from build123d import *

# Parameters (mm, degrees)
SKETCH1_W            = 694
SKETCH1_H            = 693
BOSS_EXTRUDE1_DEPTH  = 3
M6_CLEARANCE_HOLE1_D = 6.6
LPATTERN1_COUNT      = 3
LPATTERN1_PITCH      = 297
MIRROR1_COPY_1_D     = 6.6
MIRROR1_COPY_2_D     = 6.6
M6_CLEARANCE_HOLE2_D = 6.6
LPATTERN2_COUNT      = 2
LPATTERN2_PITCH      = 293
MIRROR2_COPY_1_D     = 6.6
FILLET1_R            = 10
SKETCH6_R            = 4
SKETCH6_R_2          = 5
SKETCH6_R_3          = 15
CUT_EXTRUDE1_DEPTH   = 4


with BuildPart() as part:
    # Sketch1 → Boss-Extrude1 (new body)
    with BuildSketch(Plane(origin=(0, 0, 0), x_dir=(1, 0, 0), z_dir=(0, 1, 0))):
        Rectangle(SKETCH1_W, SKETCH1_H)
    extrude(amount=BOSS_EXTRUDE1_DEPTH)

    # M6 Clearance Hole1 (through all)
    with Locations(Plane(origin=(0, 3, 0), x_dir=(1, 0, 0), z_dir=(0, 1, 0))):
        with Locations((297, -337.5)):
            m6_clearance_hole1 = Hole(M6_CLEARANCE_HOLE1_D / 2)

    # LPattern1: M6 Clearance Hole1 ×3
    with Locations(*[(-i * LPATTERN1_PITCH, 0, 0) for i in range(1, LPATTERN1_COUNT)]):
        add(m6_clearance_hole1, mode=Mode.SUBTRACT)

    # Mirror1: M6 Clearance Hole1 across plane
    add(m6_clearance_hole1.mirror(Plane.XY), mode=Mode.SUBTRACT)

    # Mirror1 copy 1 (through all)
    with Locations(Plane(origin=(-297, 3, 0), x_dir=(1, 0, 0), z_dir=(0, 1, 0))):
        with Locations((297, 337.5)):
            Hole(MIRROR1_COPY_1_D / 2)

    # Mirror1 copy 2 (through all)
    with Locations(Plane(origin=(-594, 3, 0), x_dir=(1, 0, 0), z_dir=(0, 1, 0))):
        with Locations((297, 337.5)):
            Hole(MIRROR1_COPY_2_D / 2)

    # M6 Clearance Hole2 (through all)
    with Locations(Plane(origin=(0, 3, 0), x_dir=(1, 0, 0), z_dir=(0, 1, 0))):
        with Locations((338, -146.5)):
            m6_clearance_hole2 = Hole(M6_CLEARANCE_HOLE2_D / 2)

    # LPattern2: M6 Clearance Hole2 ×2
    with Locations(*[(0, 0, -i * LPATTERN2_PITCH) for i in range(1, LPATTERN2_COUNT)]):
        add(m6_clearance_hole2, mode=Mode.SUBTRACT)

    # Mirror2: M6 Clearance Hole2 across plane
    add(m6_clearance_hole2.mirror(Plane(origin=(0, 0, 0), x_dir=(0, 0, 1), z_dir=(1, 0, 0))), mode=Mode.SUBTRACT)

    # Mirror2 copy 1 (through all)
    with Locations(Plane(origin=(0, 3, -293), x_dir=(-1, 0, 0), z_dir=(0, 1, 0))):
        with Locations((338, 146.5)):
            Hole(MIRROR2_COPY_1_D / 2)

    # Fillet1
    fillet1_edges = [part.edges().sort_by_distance(p)[0] for p in [
        (-347, 1.5, -346.5),
        (347, 1.5, -346.5),
        (347, 1.5, 346.5),
        (-347, 1.5, 346.5),
    ]]
    fillet(fillet1_edges, radius=FILLET1_R)

    # Sketch6 → Cut-Extrude1 (cut, through all)
    with BuildSketch(Plane(origin=(0, 3, 0), x_dir=(1, 0, 0), z_dir=(0, 1, 0))):
        with Locations((-337, -326.5)):
            Circle(SKETCH6_R)
        with Locations((-335, -16.5)):
            Circle(SKETCH6_R_2)
        with Locations((-335, 13.5)):
            Circle(SKETCH6_R_2)
        with Locations((-322, 183.5)):
            Circle(SKETCH6_R_3)
        with Locations((-322, 231.5)):
            Circle(SKETCH6_R_3)
        with Locations((-322, 321.5)):
            Circle(SKETCH6_R_3)
    extrude(amount=-CUT_EXTRUDE1_DEPTH, mode=Mode.SUBTRACT)


solid = part.part
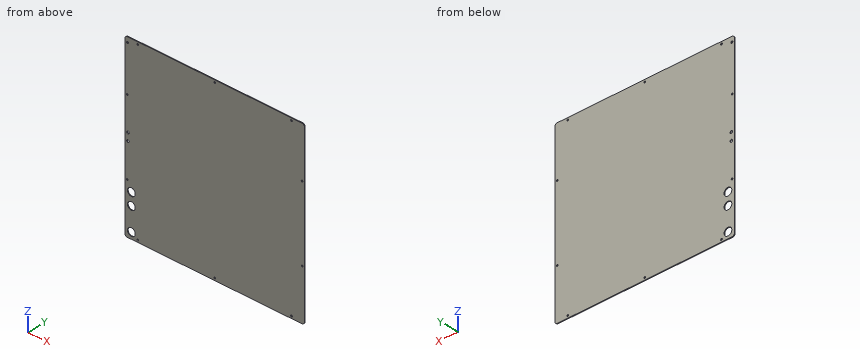
Here's how the part is built. I have some questions about the finished solid (model axes, mm). Round coordinates to 2 decimals unless told otherwise and drop trailing zeros. Write each loop counter-clockwise with the first axis right and the second up, starting at its lowest first coordinate (ties: lowest second). Pieces come first, ordered by that corner, then holes. Notation, with made-up numbers: (-19.5, 71.25) -> (-1.5, 71.25) arc R22 ccw to (-1.5, 84.25) -> close; hole circle Ø9 at (11, -17). An arc over 180 degrees is marked (long way). One line per item, written item: value.
1) Suppose I cut it at A-A on z = -321.5. List the corners of the cut face in (x, y) for me, plus the area to 3 significant figures.
Filled sheet:
outline: (-347, 0) -> (-337, 0) -> (-337, 3) -> (-347, 3) -> close; (-307, 0) -> (347, 0) -> (347, 3) -> (-307, 3) -> close
area: 1,990 mm2
2) I'm going to push a flat-ended pin straight in: pin 1 Ø5.5 at (x, z) = (338, 146.5) entering from +Y. Where does the tip first touch, or does it pass through?
Filled sheet:
pin 1: passes through
3) If I drill on line 1 (Z direction, x = -297, y = 1.1); line 2 (X direction, y = 2.1, z = 337.5); line 3 (Z direction, x = -322, y = 1.7), over which ranges is the centre line in solid material (lowest first)? Write a range as [from, to].
Filled sheet:
line 1: z = [-346.5, -340.8], [-334.2, 334.2], [340.8, 346.5]
line 2: x = [-346.95, -300.3], [-293.7, -3.3], [3.3, 293.7], [300.3, 346.95]
line 3: z = [-346.5, -336.5], [-306.5, -246.5], [-216.5, -198.5], [-168.5, 346.5]
